Build history of the part. All positions in model axes, mm. Face numbers are marked on the shaded views. A direction names the side the tool comes from. Round coordinates to 2 decimals unless told otherwise and drop trailing zeros. Write each loop counter-clockwise with the first axis right and the second up, starting at its lowest first coordinate (ties: lowest second). Pieces come first, ordered by that corner, then holes. Notation, with made-up numbers: (68.25, 13) -> (78.25, 13) arc R8 cw to (78.25, 17) -> close; hole circle Ø3 at (-2, 74.5). An arc over 180 degrees is marked (long way). Answer in a Markdown table with one row per item.
```python
from build123d import *

# Parameters (mm, degrees)
MAIN_START                  = -6.35
MAIN_BODY_EXTRUDE_OUTLINE_R = 34.544
MAIN_BODY_EXTRUDE_DEPTH     = 19.05
A_START                     = -12.7
SKETCH3_W                   = 38.1
SKETCH3_H                   = 25.4
A_ARM_CUT_EXTRUDE_DEPTH     = 12.7
SKETCH2_R                   = 39.3065
SKETCH2_R_2                 = 34.544
WHEEL_BEARING_EXTRUDE_DEPTH = 17.526
F_1_4_CLEARANCE_HOLE1_D     = 6.7564


# Read off the part's stored shape, not the designer's step: Main Body Extrude
with BuildPart() as part:
    # Main Body Extrude outline → Main Body Extrude (new body)
    with BuildSketch(Plane.XY.offset(MAIN_START)):
        with BuildLine():
            Line((27.480731972, 99.845136477), (39.047879642, 176.532662304))
            ThreePointArc((39.047879642, 176.532662304), (39.130976131, 187.677399272), (36.082648081, 198.397462855))
            Line((36.082648081, 198.397462855), (12.081280182, 252.245136477))
            Line((12.081280182, 252.245136477), (12.081280182, 277.645136477))
            Line((12.081280182, 277.645136477), (-26.018719818, 277.645136477))
            Line((-26.018719818, 277.645136477), (-26.018719818, 252.245136477))
            Line((-26.018719818, 252.245136477), (-38.372251652, 190.053187868))
            ThreePointArc((-38.372251652, 190.053187868), (-38.990928758, 179.14568581), (-36.583444609, 168.489214415))
            Line((-36.583444609, 168.489214415), (-10.619268028, 99.845136477))
            Line((-10.619268028, 99.845136477), (-10.619268028, 74.445136477))
            Line((-10.619268028, 74.445136477), (27.480731972, 74.445136477))
            Line((27.480731972, 74.445136477), (27.480731972, 99.845136477))
        make_face()
        with BuildLine():
            ThreePointArc((-25.494117557, 152.632946315), (-12.721668299, 145.266691439), (1.866319763, 143.124782188))
            Line((1.866319763, 143.124782188), (-9.153762694, 109.432323748))
            Line((-9.153762694, 109.432323748), (-25.494117557, 152.632946315))
        make_face(mode=Mode.SUBTRACT)
        Polygon((-7.391297603, 104.607636477), (3.945650004, 139.268868599), (23.044050934, 104.607636477), align=None, mode=Mode.SUBTRACT)
        with BuildLine():
            ThreePointArc((5.282813212, 143.421136093), (19.947813793, 148.420513168), (31.541530581, 158.698730145))
            Line((31.541530581, 158.698730145), (24.089008073, 109.290221793))
            Line((24.089008073, 109.290221793), (5.282813212, 143.421136093))
        make_face(mode=Mode.SUBTRACT)
        with BuildLine():
            ThreePointArc((-5.038778466, 221.353506402), (-18.844806738, 216.790174549), (-30.047186356, 207.519947737))
            Line((-30.047186356, 207.519947737), (-22.604404483, 244.989483896))
            Line((-22.604404483, 244.989483896), (-5.038778466, 221.353506402))
        make_face(mode=Mode.SUBTRACT)
        Polygon((-3.478576257, 224.576955104), (-20.501465739, 247.482636477), (7.934620863, 247.482636477), align=None, mode=Mode.SUBTRACT)
        with Locations((0.181025656, 182.395136477)):
            Circle(MAIN_BODY_EXTRUDE_OUTLINE_R, mode=Mode.SUBTRACT)
        with BuildLine():
            Line((-1.379394493, 221.670650875), (10.166551929, 244.842753057))
            Line((10.166551929, 244.842753057), (24.09762487, 213.588039906))
            ThreePointArc((24.09762487, 213.588039906), (12.067229239, 219.861376035), (-1.379394493, 221.670650875))
        make_face(mode=Mode.SUBTRACT)
    extrude(amount=MAIN_BODY_EXTRUDE_DEPTH)

    # Sketch3 → A Arm Cut Extrude (cut)
    with BuildSketch(Plane.XY.offset(12.7).offset(A_START)):
        with Locations((-6.968719818, 264.945136477)):
            Rectangle(SKETCH3_W, SKETCH3_H)
        with Locations((8.430731972, 87.145136477)):
            Rectangle(SKETCH3_W, SKETCH3_H)
    extrude(amount=A_ARM_CUT_EXTRUDE_DEPTH, mode=Mode.SUBTRACT)

    # Sketch2 → Wheel Bearing Extrude (add)
    with BuildSketch(Plane.XY.offset(12.7)):
        with Locations(Location((0.181025656, 182.395136477, 0), (0, 0, 168.765257697))):
            Circle(SKETCH2_R)
        with Locations((0.181025656, 182.395136477)):
            Circle(SKETCH2_R_2, mode=Mode.SUBTRACT)
    extrude(amount=WHEEL_BEARING_EXTRUDE_DEPTH)

    # 1/4 Clearance Hole1 (through all)
    with Locations(Plane(origin=(-16.366719818, 264.945136477, 0), x_dir=(1, 0, 0), z_dir=(0, 0, 1))):
        with Locations((0, 0), (18.796, 0), (15.39945179, -177.8), (34.19545179, -177.8)):
            Hole(F_1_4_CLEARANCE_HOLE1_D / 2)


solid = part.part
```
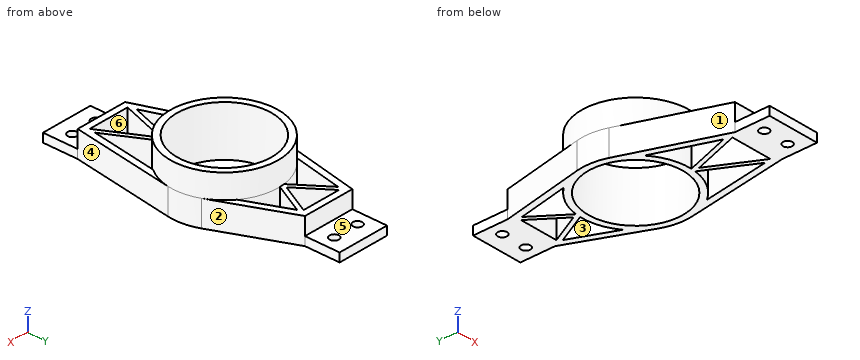
Q1. Saw through at D-D on z = 9. Write the cut outline in (x, y), plus the area to 3 significant figures.
A:
| item | result |
|---|---|
| outline | (-38.37, 190.05) arc R39.31 ccw to (-36.58, 168.49) -> (-10.62, 99.85) -> (27.48, 99.85) -> (39.05, 176.53) arc R39.31 ccw to (36.08, 198.4) -> (12.08, 252.25) -> (-26.02, 252.25) -> close; hole circle Ø69.09 at (0.18, 182.4); hole (-30.05, 207.52) arc R39.31 cw to (-5.04, 221.35) -> (-22.6, 244.99) -> close; hole (-25.49, 152.63) -> (-9.15, 109.43) -> (1.87, 143.12) arc R39.31 cw to start; hole (-20.5, 247.48) -> (-3.48, 224.58) -> (7.93, 247.48) -> close; hole (-7.39, 104.61) -> (23.04, 104.61) -> (3.95, 139.27) -> close; hole (-1.38, 221.67) arc R39.31 cw to (24.1, 213.59) -> (10.17, 244.84) -> close; hole (5.28, 143.42) -> (24.09, 109.29) -> (31.54, 158.7) arc R39.31 cw to start |
| area | 2,890 mm² |
Q2. Which spindle directions (+Z, -Z, +X, -X, +Y, -Y) get a long thin tool onto all of the face, cutting with end or side? Do the marked faces 4, 5 and 6. Say none if no direction does.
A:
| item | result |
|---|---|
| face 4 | +Z, -Z, +X, -Y |
| face 5 | +Z, +X, -X, +Y |
| face 6 | +Z, -Z |
Q3. Saw through at B-B on y = 172.5. Write the cut outline in (x, z).
A:
| item | result |
|---|---|
| outline | (-37.86, -6.35) -> (-32.92, -6.35) -> (-32.92, 30.23) -> (-37.86, 30.23) -> close; (33.28, -6.35) -> (38.44, -6.35) -> (38.44, 12.7) -> (38.22, 12.7) -> (38.22, 30.23) -> (33.28, 30.23) -> close |
Q4. Two-plate mould, pull along Y, no slides. Class the marked faces 1, 2 and 3: released by +Y, released by -Y, zero draft, split by the parting line, or undercut.
A:
| item | result |
|---|---|
| face 1 | released by -Y |
| face 2 | released by +Y |
| face 3 | undercut |
Q5. Saw through at C-C on x = -32.5. Write the cut outline in (y, z).
A:
| item | result |
|---|---|
| outline | (157.69, -6.35) -> (171.2, -6.35) -> (171.2, 30.23) -> (160.56, 30.23) -> (160.56, 12.7) -> (157.69, 12.7) -> close; (193.59, -6.35) -> (219.62, -6.35) -> (219.62, 12.7) -> (204.23, 12.7) -> (204.23, 30.23) -> (193.59, 30.23) -> close |
Q6. Wall check: line 1 (Y direction, x = 22, z = 11); line 2 (Z direction, x = -13.5, y = 109); line 3 (X direction, y = 175.5, z = -3). Give the ranges that are in metal, low to high. Write a range as [from, to].
A:
| item | result |
|---|---|
| line 1 | [99.85, 104.61], [106.5, 113.08], [149.7, 155.61], [209.18, 215.09], [218.29, 229.99] |
| line 2 | [-6.35, 12.7] |
| line 3 | [-38.52, -33.67], [34.03, 38.89] |
Q7. Drop flat-ended pins along their axis: P1, Ø10, axis at x = -11.5, z = 9.5, coming from the +Y side; P2, Ø1, axis at x = 10, y = 127, coming from the +Z side; P3, Ø5, axis at x = 8, y = 102, coming from the +Z side; P4, Ø3, axis at y = 92.5, z = -2, coming from the +X side. Give the stop position or say it passes through.
A:
| item | result |
|---|---|
| P1 | y = 252.25 |
| P2 | through |
| P3 | z = 12.7 |
| P4 | x = 27.48 |
Q8. Saw through at A-A on x = 18. Write the cut outline in (y, z), plus the area to 3 significant figures.
A:
| item | result |
|---|---|
| outline | (74.45, -6.35) -> (83.77, -6.35) -> (83.77, 0) -> (74.45, 0) -> close; (90.52, -6.35) -> (104.61, -6.35) -> (104.61, 12.7) -> (99.85, 12.7) -> (99.85, 0) -> (90.52, 0) -> close; (113.76, -6.35) -> (120.34, -6.35) -> (120.34, 12.7) -> (113.76, 12.7) -> close; (147.36, -6.35) -> (152.8, -6.35) -> (152.8, 30.23) -> (147.36, 30.23) -> close; (211.99, -6.35) -> (217.43, -6.35) -> (217.43, 30.23) -> (211.99, 30.23) -> close; (227.27, -6.35) -> (238.97, -6.35) -> (238.97, 12.7) -> (227.27, 12.7) -> close |
| area | 955 mm² |
